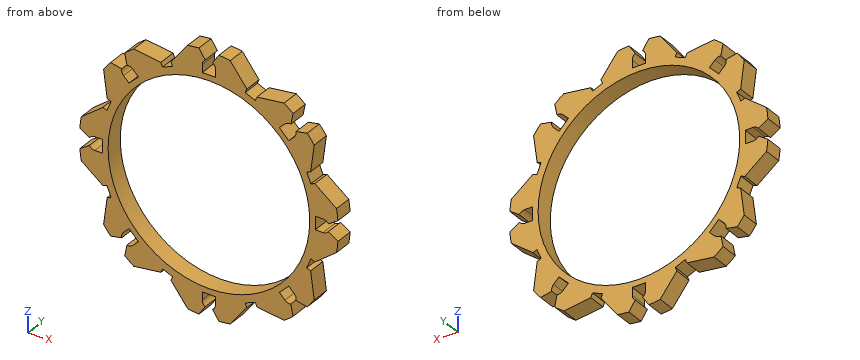
```python
from build123d import *

# Parameters (mm, degrees)
SKETCH1_R           = 54.55
BOSS_EXTRUDE1_DEPTH = 7.5
SKETCH2_R           = 42.5
CUT_EXTRUDE1_DEPTH  = 78.509063986
CUT_EXTRUDE2_DEPTH  = 78.509063986
CUT_EXTRUDE6_DEPTH  = 78.509063986
CIRPATTERN1_COUNT   = 8
CIRPATTERN2_COUNT   = 8


with BuildPart() as part:
    # Sketch1 → Boss-Extrude1 (new body)
    with BuildSketch(Plane(origin=(0, 0, 0), x_dir=(1, 0, 0), z_dir=(0, 1, 0))):
        with Locations(Location((0, 0, 0), (0, 0, 270))):
            Circle(SKETCH1_R)
    extrude(amount=BOSS_EXTRUDE1_DEPTH)

    # Sketch2 → Cut-Extrude1 (cut, through all)
    with BuildSketch(Plane(origin=(0, 7.5, 0), x_dir=(1, 0, 0), z_dir=(0, 1, 0))):
        with Locations(Location((0, 0, 0), (0, 0, 270))):
            Circle(SKETCH2_R)
    extrude(amount=-CUT_EXTRUDE1_DEPTH, mode=Mode.SUBTRACT)

    # Sketch3 → Cut-Extrude2 (cut, through all)
    with BuildSketch(Plane(origin=(0, 7.5, 0), x_dir=(1, 0, 0), z_dir=(0, 1, 0))):
        with BuildLine():
            Line((-2.8, -48.082), (-2.8, -44.832))
            Line((-2.8, -44.832), (2.8, -44.832))
            Line((2.8, -44.832), (2.8, -48.082))
            ThreePointArc((2.8, -48.082), (2.46937954, -49.401910863), (1.555596652, -50.410114914))
            Line((1.555596652, -50.410114914), (4.212915889, -54.387074197))
            ThreePointArc((4.212915889, -54.387074197), (0, -54.55), (-4.212915889, -54.387074197))
            Line((-4.212915889, -54.387074197), (-1.555596652, -50.410114914))
            ThreePointArc((-1.555596652, -50.410114914), (-2.46937954, -49.401910863), (-2.8, -48.082))
        make_face()
    cut_extrude2 = extrude(amount=-CUT_EXTRUDE2_DEPTH, mode=Mode.SUBTRACT)

    # Sketch9 → Cut-Extrude6 (cut, through all)
    with BuildSketch(Plane(origin=(0, 7.5, 0), x_dir=(1, 0, 0), z_dir=(0, 1, 0))):
        with BuildLine():
            Line((-20.257229317, -42.895088115), (-31.690865911, -44.400354929))
            ThreePointArc((-31.690865911, -44.400354929), (-20.875381236, -50.397628498), (-8.98696587, -53.804618245))
            Line((-8.98696587, -53.804618245), (-16.007383468, -44.655431904))
            Line((-16.007383468, -44.655431904), (-15.318553289, -42.992448745))
            Line((-15.318553289, -42.992448745), (-19.568399139, -41.232104956))
            Line((-19.568399139, -41.232104956), (-20.257229317, -42.895088115))
        make_face()
    cut_extrude6 = extrude(amount=-CUT_EXTRUDE6_DEPTH, mode=Mode.SUBTRACT)

    # CirPattern1: Cut-Extrude2 ×8 about axis
    cirpattern1_axis = Axis((0, 0, 0), (0, 1, 0))
    for i in range(1, CIRPATTERN1_COUNT):
        add(cut_extrude2.rotate(cirpattern1_axis, i * 360 / CIRPATTERN1_COUNT), mode=Mode.SUBTRACT)

    # CirPattern2: Cut-Extrude6 ×8 about axis
    cirpattern2_axis = Axis((0, 0, 0), (0, 1, 0))
    for i in range(1, CIRPATTERN2_COUNT):
        add(cut_extrude6.rotate(cirpattern2_axis, i * 360 / CIRPATTERN2_COUNT), mode=Mode.SUBTRACT)


solid = part.part
```
Build history of the part. All positions in model axes, mm. Coordinates: 2 decimals unless noted, no trailing zeros. Order: outer loops, then holes, each group sorted by start corner. A loop starts at its lowest first (then second) coordinate and runs counter-clockwise, first axis right, second up. Notation, with made-up numbers: (35.5, 17) -> (85.5, 17) arc R20 ccw to (85.5, 40) -> close; hole circle Ø6 at (12, -35.5). An arc over 180 degrees is marked (long way). Answer in a Markdown table with one row per item. Add a question column.
Q1. Band-saw the part on A-A, the plane z = 0. List the corners of the cut face in (x, y), then the cut area to 3 significant figures.
Q2. Band-saw the part on B-B, the plane x = 0. List the corners of the cut face in (y, z).
Q3. Drop flat-ended pins along their axis: pin 1 (1 mm diameter, centred on y = 4.5, z = 5, fed in from -X); pin 2 (1 mm diameter, centred on y = 3.5, z = 46, fed in from +X); pin 3 (1.5 mm diameter, centred on x = -38.5, y = 3.5, fed in from +Z). Give the stop position or say it passes through.
Q4. Wall check: line 1 along X through (y, z) = (2, 0); line 2 along X through (y, z) = (6.5, -34); line 3 along Z through (x, y) = (13.5, 5.5). Give the ranges that are in metal, low to high. Write a range as [from, to].
Answers follow:
| question | item | result |
|---|---|---|
| 1 | outline | (-44.83, 0) -> (-42.5, 0) -> (-42.5, 7.5) -> (-44.83, 7.5) -> close; (42.5, 0) -> (44.83, 0) -> (44.83, 7.5) -> (42.5, 7.5) -> close |
| 1 | area | 35.0 mm^2 |
| 2 | outline | (0, -44.83) -> (7.5, -44.83) -> (7.5, -42.5) -> (0, -42.5) -> close; (0, 42.5) -> (7.5, 42.5) -> (7.5, 44.83) -> (0, 44.83) -> close |
| 3 | pin 1 | x = -54.36 |
| 3 | pin 2 | x = 15.36 |
| 3 | pin 3 | z = 35.04 |
| 4 | line 1 | [-44.83, -42.5], [42.5, 44.83] |
| 4 | line 2 | [-42.66, -36.8], [-30.04, -25.5], [25.5, 30.04], [36.8, 42.66] |
| 4 | line 3 | [-47.92, -40.3], [40.3, 47.92] |
